Work out the finished part from the listing and answer in its coordinate system (mm). A direction names the side the tool comes from. Round coordinates to 2 decimals unless told otherwise and drop trailing zeros. Write each loop counter-clockwise with the first axis right and the second up, starting at its lowest first coordinate (ties: lowest second). Pieces come first, ordered by that corner, then holes. Notation, with made-up numbers: (21, 71.25) - (64, 71.25) arc R12 cw to (64, 88.25) - close; hole circle Ø4 at (-12, -7.5). An arc over 180 degrees is marked (long way). Answer as a JSON object with one key per item and string values.
Autodesk Fusion 360 part; units mm, degrees
sketch "Sketch2" plane through (0, 0, 0) normal (0, 0, 1) x (1, 0, 0)
  line L0 (-6, 6) -> (6, 6)
  line L1 (6, 6) -> (6, -6)
  line L2 (6, -6) -> (-6, -6)
  line L3 (-6, -6) -> (-6, 6)
  line L4 (-6, 6) -> (6, -6) construction
  line L5 (6, 6) -> (-6, -6) construction
  dimension "d1" = 12
  dimension "d2" = 12
extrude "Extrude1" add sketch "Sketch2" along normal blind 14 makes body 1
sketch "Sketch3" plane through (0, -6, 0) normal (0, -1, 0) x (1, 0, 0)
  line L0 (-6, 0) -> (6, 0)
  line L1 (6, 0) -> (6, 14)
  line L2 (6, 14) -> (-6, 14)
  line L3 (-6, 14) -> (-6, 0)
  line L4 (-6, 0) -> (6, 0)
  line L5 (6, 0) -> (6, -30.9661)
  line L6 (6, -30.9661) -> (-6, -30.9661)
  line L7 (-6, -30.9661) -> (-6, 0)
  line L8 (0, 0) -> (0, -30.9661) construction
  line L9 (13, -19.7077) -> (6.5, -8.4494)
  line L10 (6.5, -8.4494) -> (-6.5, -8.4494)
  line L11 (-6.5, -8.4494) -> (-13, -19.7077)
  line L12 (-13, -19.7077) -> (-6.5, -30.9661)
  line L13 (-6.5, -30.9661) -> (6.5, -30.9661)
  line L14 (6.5, -30.9661) -> (13, -19.7077)
  point P0 (0, -19.7077)
  dimension "d5" = 13
extrude "Extrude2" add sketch "Sketch3" along normal blind 17 separate body contours L5 L6 L7 L10 L13 | L7 L10 L11 L12 L13 | L5 L9 L10 L13 L14 makes body 2
extrude "Extrude3" add 1 faces at (2.1667, -6, -15.955) along direction (0, 1, 0) blind 12 on bodies 2 bodies 2
extrude "Extrude4" add 1 faces at (2, -2, 0) along direction (0, 0, -1) blind 10.3851 on bodies 1 bodies 1 2
Item 1: A cutting plane is placed at D-D (y = -18.5). Write down the section's boundary in (x, z).
Results found:
{"outline": "(-13, -19.71) - (-6.5, -30.97) - (6.5, -30.97) - (13, -19.71) - (6.5, -8.45) - (-6.5, -8.45) - close"}
Item 2: Each of these flat-tipped pins is pushed along its axis until it touches: P1, Ø13, axis at y = 2.5, z = 5, coming from the +X side; P2, Ø6, axis at x = 1, z = -1, coming from the -Y side; P3, Ø5, axis at y = -7.5, z = -9, coming from the +X side. Where does it stop, or does it pass through?
Results found:
{"P1": "x = 6", "P2": "y = -6", "P3": "x = 8.26"}
Item 3: Consider line 1 along X through (y, z) = (-1.25, -2.5); line 2 along Z through (x, y) = (-3, -17.25). Determine where each line is inside the solid, lowest interval first.
Results found:
{"line 1": "-6 to 6", "line 2": "-30.97 to -8.45"}
Item 4: A cutting plane is placed at A-A (y = -3). Write down the section's boundary in (x, z).
Results found:
{"outline": "(-13, -19.71) - (-6.5, -30.97) - (6.5, -30.97) - (13, -19.71) - (6.5, -8.45) - (6, -8.45) - (6, 14) - (-6, 14) - (-6, -8.45) - (-6.5, -8.45) - close"}
Item 5: A cutting plane is placed at C-C (z = 11.5). Write down the section's boundary in (x, y), and give its area (3 significant figures).
Results found:
{"outline": "(-6, -6) - (6, -6) - (6, 6) - (-6, 6) - close", "area": "144 mm²"}
Item 6: For faces 1 (the flat face through (-6, 0, 3)), 2 (the flat face through (0, 6, -9)), 3 (the flat face through (6, 0, 3)), 4 (the flat face through (0, -6, 3)), determine the directions among +Z, -Z, +X, -X, +Y, -Y from which every point of the face is accessible in a straight line to the end or side of a thin tool.
Results found:
{"face 1": "+Z, -X, +Y, -Y", "face 2": "+Z, -Z, +X, -X, +Y", "face 3": "+Z, +X, +Y, -Y", "face 4": "+Z, +X, -X, -Y"}
Item 7: A cutting plane is placed at B-B (x = -4.75). Write down the section's boundary in (y, z), and give its area (3 significant figures).
Results found:
{"outline": "(-23, -30.97) - (6, -30.97) - (6, 14) - (-6, 14) - (-6, -8.45) - (-23, -8.45) - close", "area": "922 mm²"}
